The figure shows three views and two pictorial views of one solid part (mm, origin at its lowest corner). Answer the questions. A direction names the side the tool comes from. Give positions to 0.01 mm unless a question says otherwise; leave off trailing zeros. Write each loop counter-clockwise with the first axis right and the second up, starting at its lowest first coordinate (ties: lowest second). Pieces come first, ordered by that corner, then holes. Notation, with made-up numbers: (10, 74) -> (69, 74) arc R10 ccw to (69, 93) -> close; hole circle Ø2 at (-15.75, -39). An arc over 180 degrees is marked (long way). Use a Markdown table: item, result.
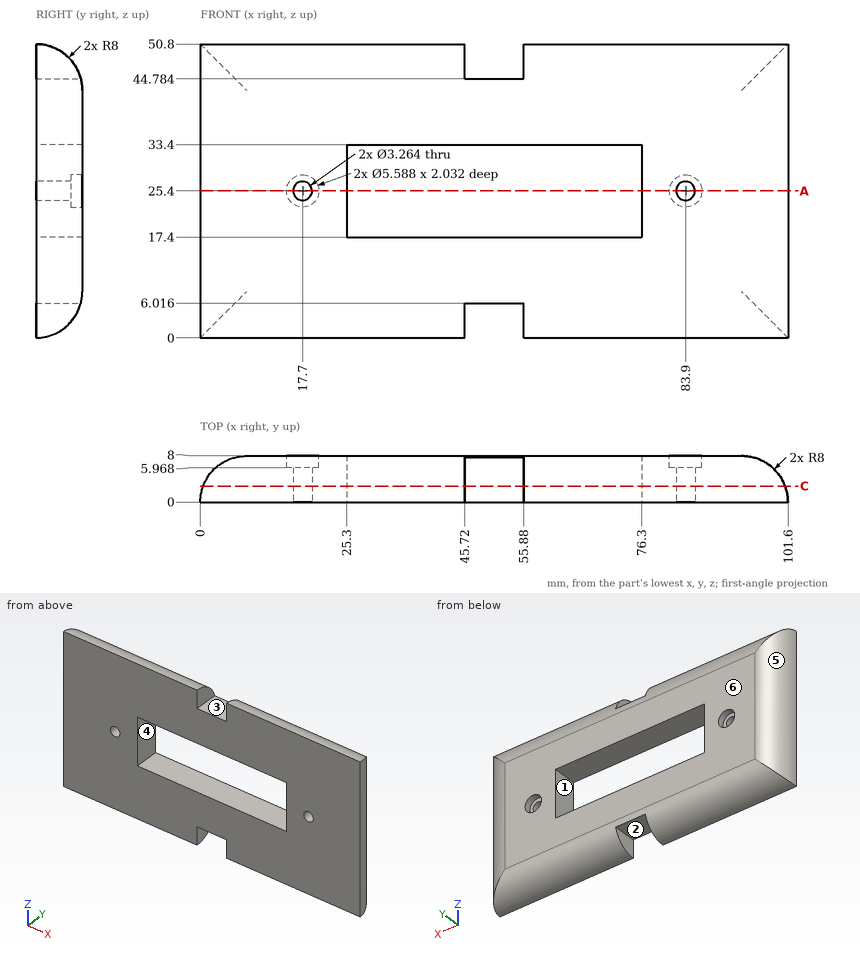
Item 1: A cutting plane is placed at C-C (y = 2.75). Give the vertices of the cut face in (x, z), then the cut area to 3 significant figures.
Return value:
| item | result |
|---|---|
| outline | (0.49, 0.49) -> (45.72, 0.49) -> (45.72, 6.02) -> (55.88, 6.02) -> (55.88, 0.49) -> (101.11, 0.49) -> (101.11, 50.31) -> (55.88, 50.31) -> (55.88, 44.78) -> (45.72, 44.78) -> (45.72, 50.31) -> (0.49, 50.31) -> close; hole circle Ø3.26 at (17.7, 25.4); hole (25.3, 17.4) -> (76.3, 17.4) -> (76.3, 33.4) -> (25.3, 33.4) -> close; hole circle Ø3.26 at (83.9, 25.4) |
| area | 4,070 mm^2 |
Item 2: Straight lines are drawn through the part: line 1 along X through (y, z) = (1.6, 25.4); line 2 along X through (y, z) = (6.8, 25.4) (1 decimal); line 3 along Z through (x, y) = (53, 4.25). For each, find the intervals that lie inside material, in ascending order. Write a range as [from, to].
Return value:
| item | result |
|---|---|
| line 1 | [0.16, 16.07], [19.33, 25.3], [76.3, 82.27], [85.53, 101.44] |
| line 2 | [3.8, 14.9], [20.5, 25.3], [76.3, 81.1], [86.7, 97.8] |
| line 3 | [6.02, 17.4], [33.4, 44.78] |
Item 3: A tool of negligible diameter and unlimited length cuts with its end or side. For the marked faces 1, 2 and 3, from which of +Z, -Z, +X, -X, +Y, -Y can it reach the whole face along a straight path? Write none if from no direction.
Return value:
| item | result |
|---|---|
| face 1 | +Y, -Y |
| face 2 | -Z, +Y, -Y |
| face 3 | +Z, +Y, -Y |
Item 4: Each of these flat-tipped pins is pushed along its axis until it touches: P1, Ø2.5, axis at x = 43, y = 5, coming from the -Z side; P2, Ø4, axis at x = 83.9, z = 25.4, coming from the +Y side; P3, Ø2, axis at y = 5, z = 29, coming from the +X side. Where does it stop, or does it pass through?
Return value:
| item | result |
|---|---|
| P1 | z = 0.93 |
| P2 | y = 5.97 |
| P3 | x = 100.53 |
Item 5: For a pull along X with two mould halves and no side action, classify the marked faces 4, 5 and 6 as +X half, -X half, draft (parallel to the pull), parting line (faces both ways), or undercut.
Return value:
| item | result |
|---|---|
| face 4 | undercut |
| face 5 | -X half |
| face 6 | draft |
Item 6: A cutting plane is placed at A-A (z = 25.4). Count the separate pieces of the cut face and the enclosed holes in it, then the cut area to 3 significant figures.
Return value:
| item | result |
|---|---|
| separate pieces | 4 |
| enclosed holes | 0 |
| area | 316 mm^2 |
